Design review of the part shown in the three views and the two pictorial views. Dimensions are in mm from the part's minimum x, y and z. Coordinates: 2 decimals unless noted, no trailing zeros. Loops run counter-clockwise (first coordinate to the right, second up) from the corner with the lowest first, then second, coordinate; pieces in that order, holes last. Notation, with made-up numbers: M -36,-9.5 L 17,-9.5 A24 ccw 17,2.5 Z; hole C -1,9.5 d10. An arc over 180 degrees is marked long. Answer as a JSON object with one key per item and string values. Group by question number.
Item 1: Add section D-D (x = 11.5). State the section outline as (y, z) points.
Item 2: Insertion check: pin 1 (1 mm diameter, centred on y = 3, z = 1, fed in from -X); pin 2 (4 mm diameter, centred on y = 8.5, z = 8, fed in from +X); pin 3 (1.5 mm diameter, centred on y = 2.5, z = 2, fed in from -X). Each pin has a flat end and moves straight along its axis. Give the tip position at first contact, or say it passes through.
Item 3: Add section C-C (x = 4). State the section outline as (y, z) points (1 decimal), then the cut area to 3 significant figures.
Item 4: Mouldability with a two-part tool opening along Y and no side actions: class the marked faces 1, 2 and 3 as +Y half, -Y half, draft (parallel to the pull), parting line (faces both ways), or undercut.
Item 5: Add section B-B (z = 3.75). State the section outline as (x, y) points.
Item 6: Wall thickness on L1, parallel to Y at x = 7, z = 7.5; L2, parallel to X at y = 3.75, z = 3 (1 decimal); L3, parallel to Z at x = 8.25, y = 9.5: over which ranges is each line inside the solid? List them lowest first. Write a range as from..to.
Item 7: Add section A-A (y = 5). State the section outline as (x, z) points (1 decimal).
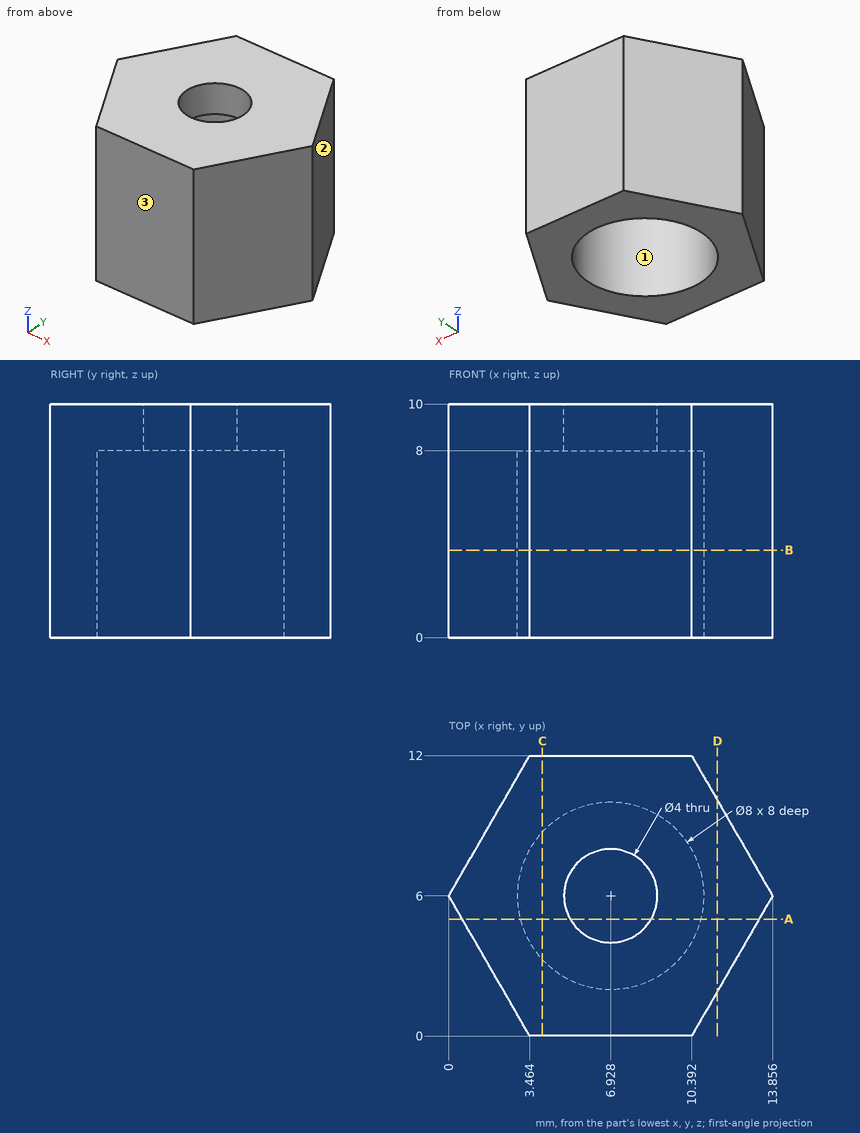
From the geometry:
{
 "1": {"outline": "M 1.92,0 L 10.08,0 L 10.08,10 L 1.92,10 Z"},
 "2": {"pin 1": "stops at x = 1.44", "pin 2": "stops at x = 13.57", "pin 3": "stops at x = 1.59"},
 "3": {"outline": "M 0,0 L 3.3,0 L 3.3,8 L 8.7,8 L 8.7,0 L 12,0 L 12,10 L 0,10 Z", "area": "76.4 mm²"},
 "4": {"face 1": "undercut", "face 2": "+Y half", "face 3": "-Y half"},
 "5": {"outline": "M 0,6 L 3.46,0 L 10.39,0 L 13.86,6 L 10.39,12 L 3.46,12 Z; hole C 6.93,6 d8"},
 "6": {"L1": "y = 0..2, 10..12", "L2": "x = 1.3..3.6, 10.2..12.6", "L3": "z = 8..10"},
 "7": {"outline": "M 0.6,0 L 3.1,0 L 3.1,8 L 5.2,8 L 5.2,10 L 0.6,10 Z; M 8.7,8 L 10.8,8 L 10.8,0 L 13.3,0 L 13.3,10 L 8.7,10 Z"}
}
